CAD build for the part. Positions are in the model's coordinates, mm. Coordinates: 2 decimals unless noted, no trailing zeros. Loops run counter-clockwise (first coordinate to the right, second up) from the corner with the lowest first, then second, coordinate; pieces in that order, holes last. Notation, with made-up numbers: (11, 14) -> (17, 14) arc R30 cw to (17, 48) -> close; hole circle Ø1 at (-14, -35.5). An arc over 180 degrees is marked (long way). Answer as CSV lines item,"result". Start each with the question number.
```python
from build123d import *

# Parameters (mm, degrees)
CURVED_PLATE_DEPTH   = 50.8
SKETCH3_R            = 3.5687
MOUNTING_HOLES_DEPTH = 66.75


with BuildPart() as part:
    # Sketch1 → Curved Plate (new body)
    with BuildSketch(Plane(origin=(0, 0, 0), x_dir=(1, 0, 0), z_dir=(0, 1, 0))):
        with BuildLine():
            Line((170.139573777, 0), (175, 0))
            ThreePointArc((175, 0), (0, 65.75), (-175, 0))
            Line((-175, 0), (-170.139573777, 0))
            ThreePointArc((-170.139573777, 0), (0, 62.575), (170.139573777, 0))
        make_face()
    extrude(amount=CURVED_PLATE_DEPTH)

    # Sketch3 → Mounting Holes (cut, through all)
    with BuildSketch(Plane.XY):
        with Locations((-159.125, 25.4)):
            Circle(SKETCH3_R)
        with Locations((159.125, 25.4)):
            Circle(SKETCH3_R)
    extrude(amount=-MOUNTING_HOLES_DEPTH, mode=Mode.SUBTRACT)


solid = part.part
```
Q1. Pin check, flat tips, straight feed: pin 1 Ø8 at (x, y) = (38.5, 20) entering from -Z; pin 2 Ø4 at (y, z) = (45, -31) entering from +X; pin 3 Ø11.5 at (x, y) = (-159.125, 25.4) entering from -Z. Stop position of each tip, or through.
Q2. Saw through at B-B (z = -31.5). List the corners of the cut face in (x, y), and give its area (3 significant figures).
Q3. Probe probe 1 along X at (y, z) = (48, -28); probe 2 along X at (y, z) = (25, -9); probe 3 along Z at (x, y) = (-130, 19). List the from-to ranges inside material, lowest first. Write a range as from..to.
Q4. Two-plate mould, pull along Y, no slides. Class faces 1 (the cylindrical face through (-157.21, 28.41, -10.72)), 2 (the flat face through (-27, 0, -62)), 3 (the flat face through (-27, 50.8, -62)), 4 (the cylindrical face through (161.04, 28.41, -10.72)): pulls with the +Y half, pulls with the -Y half, needs draft (parallel to the pull), parting line crosses it, or undercut.
Q5. Saw through at A-A (y = 25.4). List the corners of the cut face in (x, z), and give its area (3 significant figures).
Q6. Saw through at C-C (y = 46). List the corners of the cut face in (x, z), and give its area (3 significant figures).
Q7. Saw through at D-D (z = -49.5). List the corners of the cut face in (x, y).
Ans:
1,pin 1,"stops at z = -63.5"
1,pin 2,"stops at x = 134.84"
1,pin 3,"stops at z = -17.03"
2,outline,"(-130.51, 0) -> (-123.91, 0) -> (-123.91, 50.8) -> (-130.51, 50.8) -> close; (123.91, 0) -> (130.51, 0) -> (130.51, 50.8) -> (123.91, 50.8) -> close"
2,area,"670 mm²"
3,probe 1,"x = -136.53..-130.24, 130.24..136.53"
3,probe 2,"x = -164.15..-162.67, 162.67..164.15"
3,probe 3,"z = -31.78..-28.14"
4,face 1,"undercut"
4,face 2,"pulls with the -Y half"
4,face 3,"pulls with the +Y half"
4,face 4,"undercut"
5,outline,"(-175, 0) arc R265.76 ccw to (-162.69, -10.13) -> (-162.69, -6.1) arc R262.59 cw to (-170.14, 0) -> close; (-155.56, -15.47) arc R265.76 ccw to (155.56, -15.47) -> (155.56, -11.54) arc R262.59 cw to (-155.56, -11.54) -> close; (162.69, -10.13) arc R265.76 ccw to (175, 0) -> (170.14, 0) arc R262.59 cw to (162.69, -6.1) -> close"
5,area,"1,140 mm²"
6,outline,"(-175, 0) arc R265.76 ccw to (175, 0) -> (170.14, 0) arc R262.59 cw to (-170.14, 0) -> close"
6,area,"1,190 mm²"
7,outline,"(-91.51, 0) -> (-81.83, 0) -> (-81.83, 50.8) -> (-91.51, 50.8) -> close; (81.83, 0) -> (91.51, 0) -> (91.51, 50.8) -> (81.83, 50.8) -> close"
